from build123d import *

# Parameters (mm, degrees)
F2_R     = 2.413
F3_DEPTH = 25.4
F4_DEPTH = 50.8
F5_DEPTH = 38.1
F8_SIZE  = 6.35


with BuildPart() as f1:
    # F0 (on Front) → F1 (revolve)
    with BuildSketch(Plane.XZ):
        Polygon((0, 0), (15.875, 0), (15.875, 25.4), (25.4, 25.4), (25.4, 31.75), (47.625, 31.75), (47.625, 38.1), (25.4, 38.1), (25.4, 44.45), (28.9087127894, 44.45), (47.625, 44.45), (47.625, 88.9), (0, 88.9), align=None)
    revolve(axis=Axis((0, 0, 44.45), (0, 0, -1)))

    # F2 (on face) → F3 (cut)
    with BuildSketch(Plane.XY.offset(88.9)):
        with BuildLine():
            ThreePointArc((47.625, 0), (46.9391314035, 8.0534817368), (44.9012806053, 15.875))
            Line((44.9012806053, 15.875), (31.75, 15.875))
            ThreePointArc((31.75, 15.875), (22.7697438789, 12.1552561211), (19.05, 3.175))
            Line((19.05, 3.175), (19.05, -9.1654355234))
            ThreePointArc((19.05, -9.1654355234), (22.8783240869, -23.4529355234), (33.3375, -33.9121114365))
            Line((33.3375, -33.9121114365), (33.4009492811, -33.9487438961))
            ThreePointArc((33.4009492811, -33.9487438961), (43.9252822103, -18.4040812795), (47.625, 0))
        make_face()
        with Locations((31.75, -12.7)):
            Circle(F2_R, mode=Mode.SUBTRACT)
        with Locations((31.75, 3.175)):
            Circle(F2_R, mode=Mode.SUBTRACT)
        with BuildLine():
            Line((-6.35, 47.1997682727), (-6.35, -10.9985226281))
            Line((-6.35, -10.9985226281), (0, -14.6646968374))
            Line((0, -14.6646968374), (6.35, -10.9985226281))
            Line((6.35, -10.9985226281), (6.35, 47.1997682727))
            ThreePointArc((6.35, 47.1997682727), (0, 47.625), (-6.35, 47.1997682727))
        make_face()
        with BuildLine():
            ThreePointArc((-33.3375, -33.9121114365), (-22.8783240869, -23.4529355234), (-19.05, -9.1654355234))
            Line((-19.05, -9.1654355234), (-19.05, 3.175))
            ThreePointArc((-19.05, 3.175), (-22.7697438789, 12.1552561211), (-31.75, 15.875))
            Line((-31.75, 15.875), (-44.9012806053, 15.875))
            ThreePointArc((-44.9012806053, 15.875), (-46.4048614399, -10.711183863), (-33.4009492811, -33.9487438961))
            Line((-33.4009492811, -33.9487438961), (-33.3375, -33.9121114365))
        make_face()
        with Locations((-31.75, -12.7)):
            Circle(F2_R, mode=Mode.SUBTRACT)
        with Locations((-31.75, 3.175)):
            Circle(F2_R, mode=Mode.SUBTRACT)
        with BuildLine():
            Line((0, -14.6646968374), (-6.35, -18.3308710468))
            Line((-6.35, -18.3308710468), (-6.35, -22.225))
            ThreePointArc((-6.35, -22.225), (0, -15.875), (6.35, -22.225))
            Line((6.35, -22.225), (6.35, -18.3308710468))
            Line((6.35, -18.3308710468), (0, -14.6646968374))
        make_face()
        Polygon((6.35, -10.9985226281), (0, -14.6646968374), (6.35, -18.3308710468), align=None)
        Polygon((-6.35, -10.9985226281), (-6.35, -18.3308710468), (0, -14.6646968374), align=None)
        with Locations((-31.75, 3.175)):
            Circle(F2_R)
        with Locations((-31.75, -12.7)):
            Circle(F2_R)
        with Locations((31.75, -12.7)):
            Circle(F2_R)
        with Locations((31.75, 3.175)):
            Circle(F2_R)
    extrude(amount=-F3_DEPTH, mode=Mode.SUBTRACT)

    # F2 (on face) → F4 (cut)
    with BuildSketch(Plane.XY.offset(88.9)):
        with BuildLine():
            ThreePointArc((6.35, -22.225), (0, -15.875), (-6.35, -22.225))
            Line((-6.35, -22.225), (6.35, -22.225))
        make_face()
        with BuildLine():
            Line((-6.35, -22.225), (-6.35, -47.1997682727))
            ThreePointArc((-6.35, -47.1997682727), (0, -47.625), (6.35, -47.1997682727))
            Line((6.35, -47.1997682727), (6.35, -22.225))
            Line((6.35, -22.225), (-6.35, -22.225))
        make_face()
    extrude(amount=-F4_DEPTH, mode=Mode.SUBTRACT)

    # F2 (on face) → F5 (cut)
    with BuildSketch(Plane.XY.offset(88.9)):
        with Locations((-31.75, 3.175)):
            Circle(F2_R)
        with Locations((-31.75, -12.7)):
            Circle(F2_R)
        with Locations((31.75, 3.175)):
            Circle(F2_R)
        with Locations((31.75, -12.7)):
            Circle(F2_R)
    extrude(amount=-F5_DEPTH, mode=Mode.SUBTRACT)

    # F8
    f8_edges = [f1.edges().sort_by_distance(p)[0] for p in [
        (20.950702, -42.76925, 88.9),
        (-20.950702, -42.76925, 88.9),
        (-30.033044, 36.96156, 88.9),
        (30.033044, 36.96156, 88.9),
    ]]
    chamfer(f8_edges, length=F8_SIZE)


solid = f1.part
Design review of the part built by this model. Coordinates are the model's own, in mm. A direction names the side the tool comes from. Coordinates: 2 decimals unless noted, no trailing zeros. Loops run counter-clockwise (first coordinate to the right, second up) from the corner with the lowest first, then second, coordinate; pieces in that order, holes last. Notation, with made-up numbers: M 81,40 L 113,40 A10 ccw 113,46 Z; hole C 48.5,-2.5 d2. An arc over 180 degrees is marked long. Use one line per item in the form item = value.
(1) Consider section D-D (y = -32.5). Give the number of separate pieces and of enclosed holes in the cut face, and give its area (3 significant figures).
Return value:
separate_pieces = 3
enclosed_holes = 0
area = 2,760 mm2
(2) Clearance check with flat-ended pins moving along their axes: P1, Ø2, axis at y = -1.5, z = 79.5, coming from the -X side; P2, Ø1.4, axis at x = 32.5, y = 2.5, coming from the +Z side; P3, Ø6.5, axis at x = 37, z = 75.5, coming from the -Y side (3 decimals). State where each tip first meets the part, or that it passes through.
Return value:
P1 = -19.05
P2 = 50.8
P3 = 15.875
(3) Consider section B-B (z = 57). Write out the cut boundary in (x, y) (3 decimals).
Return value:
outline = M -6.35,-47.2 L -6.35,-22.225 A6.35 cw 6.35,-22.225 L 6.35,-47.2 A47.625 ccw long Z; hole C -31.75,-12.7 d4.826; hole C -31.75,3.175 d4.826; hole C 31.75,-12.7 d4.826; hole C 31.75,3.175 d4.826
(4) For faces 1 (the face through (-34, -3, 63.5)), 2 (the face through (-32, 3, 50.8)), 3 (the face through (-1.03, 25.38, 41.32)), 4 (the face through (-3.441, 15.497, 12.878)), list the 3-axis set-ups (+Z, -Z, +X, -X, +Y, -Y) from which the entire face can be reached by the end or side of a thin tool; tool diameter is ignored.
Return value:
face_1 = +Z, -X
face_2 = +Z
face_3 = none
face_4 = -Z
(5) Consider section C-C (x = 0). Write out the cut boundary in (y, z) (3 decimals), and give its area (3 significant figures).
Return value:
outline = M -47.625,31.75 L -25.4,31.75 L -25.4,25.4 L -15.875,25.4 L -15.875,0 L 15.875,0 L 15.875,25.4 L 25.4,25.4 L 25.4,31.75 L 47.625,31.75 L 47.625,38.1 L 25.4,38.1 L 25.4,44.45 L 47.625,44.45 L 47.625,63.5 L -15.875,63.5 L -15.875,38.1 L -47.625,38.1 Z
area = 3,210 mm2
(6) Draft analysis for pull direction X (two halves, no side actions). For faces 5 (the face through (26.856, 33.575, 87.181)), 6 (the face through (-22.98, -23.63, 76.38)), 7 (the face through (34.05, 3.9, 57.24)), state which applies: pulls with the +X half, pulls with the -X half, needs draft (parallel to the pull), parting line crosses it, or undercut.
Return value:
face_5 = pulls with the +X half
face_6 = pulls with the -X half
face_7 = undercut
(7) For line 1 along Z through (x, y) = (-26, -23); line 2 along Y through (x, z) = (-31.75, 53.5); line 3 along Y through (x, z) = (31, 54), list the stretches that pass through material, from the lowest coordinate up. Write a range as from..to.
Return value:
line_1 = 31.75..38.1, 44.45..63.5
line_2 = -35.5..-15.11, -10.29..0.76, 5.59..35.5
line_3 = -36.15..-14.99, -10.41..0.88, 5.47..36.15
